Geometry check sheet. Reference: the model listing, model coordinates, mm. Give positions to 0.01 mm unless a question says otherwise; leave off trailing zeros. Loops run counter-clockwise (first coordinate to the right, second up) from the corner with the lowest first, then second, coordinate; pieces in that order, holes last. Notation, with made-up numbers: (-20, 47) -> (29, 47) arc R33 cw to (29, 85) -> close; hole circle Ø2 at (24, 85). An arc over 180 degrees is marked (long way). Write item = value, one per line.
```python
from build123d import *

# Parameters (mm, degrees)
F0_R     = 20
F0_R_2   = 10.1
F1_DEPTH = 25
F2_SIZE2 = 1.4
F2_SIZE  = 1.4
F3_SIZE2 = 1
F3_SIZE  = 1


with BuildPart() as f1:
    # F0 (on Front) → F1 (new body, symmetric)
    with BuildSketch(Plane.XZ):
        Circle(F0_R)
        Circle(F0_R_2, mode=Mode.SUBTRACT)
    extrude(amount=F1_DEPTH, both=True)

    # F2
    f2_edges = [f1.edges().sort_by_distance(p)[0] for p in [
        (-20, -25, 0),
        (-10.1, -25, 0),
    ]]
    chamfer(f2_edges, length=F2_SIZE, length2=F2_SIZE2)

    # F3
    f3_edges = [f1.edges().sort_by_distance(p)[0] for p in [
        (-10.1, 25, 0),
        (-20, 25, 0),
    ]]
    chamfer(f3_edges, length=F3_SIZE, length2=F3_SIZE2)


solid = f1.part
```
Item 1: Section check A-A, the plane z = 0. Record the cut outline in (x, y), plus the area to 3 significant figures.
Answer:
outline = (-20, -23.6) -> (-18.6, -25) -> (-11.5, -25) -> (-10.1, -23.6) -> (-10.1, 24) -> (-11.1, 25) -> (-19, 25) -> (-20, 24) -> close; (10.1, -23.6) -> (11.5, -25) -> (18.6, -25) -> (20, -23.6) -> (20, 24) -> (19, 25) -> (11.1, 25) -> (10.1, 24) -> close
area = 984 mm^2
Item 2: Section check B-B, the plane x = 0. Record the cut outline in (y, z).
Answer:
outline = (-25, -18.6) -> (-23.6, -20) -> (24, -20) -> (25, -19) -> (25, -11.1) -> (24, -10.1) -> (-23.6, -10.1) -> (-25, -11.5) -> close; (-25, 11.5) -> (-23.6, 10.1) -> (24, 10.1) -> (25, 11.1) -> (25, 19) -> (24, 20) -> (-23.6, 20) -> (-25, 18.6) -> close
Item 3: Section check C-C, the plane y = 14. Record the cut outline in (x, z).
Answer:
outline = circle Ø40 at (0, 0); hole circle Ø20.2 at (0, 0)
Item 4: Draft check along X on faces 1 (the cylindrical face through (9.634, 0.533, 3.034)), 2 (the cylindrical face through (-4.336, -0.133, -19.524)), 3 (the flat face through (8, 25, -8)). Enter one of: +X half, -X half, draft (parallel to the pull), parting line (faces both ways), or undercut.
Answer:
face_1 = undercut
face_2 = parting line
face_3 = draft
Item 5: Gauge pin test, flat ends, axial feed: pin 1 (2 mm diameter, centred on x = 11, y = -11, fed in from +Z); pin 2 (18 mm diameter, centred on x = 0, z = 0, fed in from +Y); pin 3 (1.5 mm diameter, centred on y = -17.5, z = 15, fed in from -X); pin 4 (2 mm diameter, centred on x = -8.5, y = -7.5, fed in from +Z). Record the tip position at first contact, or that the pin passes through.
Answer:
pin_1 = 17.32
pin_2 = through
pin_3 = -14.03
pin_4 = 18.54
Item 6: Thickness scan on L1, parallel to Z at x = 0, y = -13; L2, parallel to Z at x = 8, y = 14. Record the ranges inside material, lowest first. Write a range as [from, to].
Answer:
L1 = [-20, -10.1], [10.1, 20]
L2 = [-18.33, -6.17], [6.17, 18.33]
